Read the model definition and answer for the solid it produces. Units are mm, in the model's axes. A direction names the side the tool comes from. Coordinates: 2 decimals unless noted, no trailing zeros. Write each loop counter-clockwise with the first axis right and the second up, starting at its lowest first coordinate (ties: lowest second). Pieces come first, ordered by that corner, then holes. Notation, with made-up numbers: (-39, 77) - (6, 77) arc R15 cw to (6, 98) - close; hole circle Ø2 at (69, -3.5). An arc over 180 degrees is marked (long way). Return JSON: item names as keys, results as strings.
Solid Edge part; units mm, degrees
sketch "Sketch1" plane through (0, 0, 0) normal (0, 0, 1) x (1, 0, 0)
  line L0 (0, 3.1011) -> (0, 18.3411)
  line L1 (0, 18.3411) -> (22.225, 18.3411)
  line L2 (22.225, 18.3411) -> (22.225, 3.1011)
  line L3 (22.225, 3.1011) -> (0, 3.1011)
extrude "Protrusion1" add sketch "Sketch1" along normal blind 3.175
sketch "Sketch2" plane through (14.2875, 8.8161, 3.175) normal (0, 0, 1) x (1, 0, 0)
  line L0 (4.8619, -5.715) -> (7.9375, -2.6394)
  line L1 (7.9375, -5.715) -> (7.9375, -2.6394)
  line L2 (4.8619, -5.715) -> (7.9375, -5.715)
  line L3 (-14.2875, -5.715) -> (-14.2875, -0.9525)
  line L4 (-14.2875, -0.9525) -> (3.4925, -0.9525)
  line L5 (3.4925, -0.9525) -> (3.4925, -5.715)
  line L6 (3.4925, -5.715) -> (-14.2875, -5.715)
  dimension "D1" = 14.2875
  dimension "D2" = 3.4925
extrude "Cutout1" cut sketch "Sketch2" against normal through all
hole "Hole_2" at (9.525, 13.1023, 3.175) direction (0, 0, -1) diameter 3.175 end up to next
fillet "Round_5" radius 6.35 1 edges at (22.225, 18.3411, 1.5875)
(1) A cutting plane is placed at D-D (x = 3). Determine the outline of the cut face in (y, z) (3 decimals).
Answer:
{"outline": "(7.864, 0) - (18.341, 0) - (18.341, 3.175) - (7.864, 3.175) - close"}
(2) Determine the mould class of faces 3 (the face through (8.559, 14.362, 1.61)), 4 (the face through (9, 7.864, 2)), 5 (the face through (11.3, 12.5, 0)) for opening direction Y: +Y half, -Y half, draft (parallel to the pull), parting line (faces both ways), or undercut.
Answer:
{"face 3": "undercut", "face 4": "-Y half", "face 5": "draft"}
(3) Flat-ended cylindrical pins translate along their axes: P1, Ø1, axis at x = 7.5, z = 1.5, coming from the -Y side; P2, Ø1, axis at y = 4.5, z = 2.5, coming from the -X side. Find the tip coordinate at first contact, or state that the pin passes through.
Answer:
{"P1": "y = 7.86", "P2": "x = 17.78"}
(4) A cutting plane is placed at B-B (y = 11.75). Determine the outline of the cut face in (x, z) (3 decimals).
Answer:
{"outline": "(0, 0) - (8.693, 0) - (8.693, 3.175) - (0, 3.175) - close; (10.357, 0) - (22.225, 0) - (22.225, 3.175) - (10.357, 3.175) - close"}
(5) A cutting plane is placed at A-A (x = 9.75). Determine the outline of the cut face in (y, z) (3 decimals).
Answer:
{"outline": "(7.864, 0) - (11.531, 0) - (11.531, 3.175) - (7.864, 3.175) - close; (14.674, 0) - (18.341, 0) - (18.341, 3.175) - (14.674, 3.175) - close"}
(6) Straight lines are drawn through the part: line 1 (Y direction, x = 6, z = 0.3); line 2 (X direction, y = 11.75, z = 1.1) (3 decimals); line 3 (Y direction, x = 10.25, z = 0.45). For each, find the intervals that lie inside material, in ascending order. Write a range as from..to.
Answer:
{"line 1": "7.86..18.34", "line 2": "0..8.693, 10.357..22.225", "line 3": "7.86..11.69, 14.51..18.34"}
(7) Which of the six approach directions +Z, -Z, +X, -X, +Y, -Y give full straight-line access (tool end or side, diameter ignored) to faces 1 (the face through (0, 13, 2)), 2 (the face through (17.78, 6, 2))?
Answer:
{"face 1": "+Z, -Z, -X, +Y, -Y", "face 2": "+Z, -Z, -X, -Y"}
